```python
from build123d import *

# Parameters (mm, degrees)
F0_W         = 20
F0_H         = 47.7648153901
F1_DEPTH     = 3
F3_W         = 20
F3_H         = 23
F4_DEPTH     = 1.5
F5_T1_DEPTH  = 30.2867319519
F6_W         = 20
F6_H         = 2.1213203436
F7_DEPTH     = 7
F8_W         = 23.5785972327
F8_H         = 18.0557984859
F9_DEPTH     = 0.828
F10_SIZE     = 3
F11_R        = 2
F12_W        = 20
F12_H        = 16
F13_DEPTH    = 6
F14_T4_DEPTH = 61.5019292892
F14_T9_DEPTH = 61.5019292892
F15_R        = 2
F16_R        = 1
F17_W        = 2
F17_H        = 2
F18_DEPTH    = 3


# Not quite as in the source:
# - a fillet or chamfer that OpenCascade refuses, or shapes differently, is made with other operations: its cross-section is extruded or revolved along the edge and cut away or added


with BuildPart() as f1:
    # F0 (on Top) → F1 (new body)
    with BuildSketch(Plane.XY):
        Rectangle(F0_W, F0_H)
    extrude(amount=F1_DEPTH)

    # F3 (on offset) → F4 (join)
    with BuildSketch(Plane.XZ.offset(23.8824076951)):
        with Locations((0, -8.5)):
            Rectangle(F3_W, F3_H)
    extrude(amount=F4_DEPTH)

    # F5: chamfer of 2 on 1 edges, made by hand

    # F5_s2 → F5_t1 (cut)
    with BuildSketch(Plane.YZ.offset(-15.1433659759)):
        Polygon((-25.3824076951, -18), (-23.3824076951, -20), (-25.3824076951, -20), align=None)
    extrude(amount=F5_T1_DEPTH, mode=Mode.SUBTRACT)

    # F6 (on face) → F7 (join)
    with BuildSketch(Plane(origin=(0, -21.6912038475, -21.6912038475), x_dir=(1, 0, 0), z_dir=(0, -0.7071067812, -0.7071067812))):
        with Locations((0, 4.1594903709)):
            Rectangle(F6_W, F6_H)
    extrude(amount=F7_DEPTH)

    # F8 (on face) → F9 (cut)
    with BuildSketch(Plane(origin=(0, -2.1912038475, 2.1912038475), x_dir=(-1, 0, 0), z_dir=(0, 0.7071067812, -0.7071067812))):
        with Locations((-0.010414049, -33.0743109807)):
            Rectangle(F8_W, F8_H)
    extrude(amount=-F9_DEPTH, mode=Mode.SUBTRACT)

    # F10
    f10_edges = [f1.edges().sort_by_distance(p)[0] for p in [
        (-10, -29.874897, -23.407005),
        (10, -29.874897, -23.407005),
    ]]
    chamfer(f10_edges, length=F10_SIZE)

    # F11
    f11_edges = [f1.edges().sort_by_distance(p)[0] for p in [
        (0, -23.882408, 0),
        (0, -25.382408, -18),
        (0, -23.882408, -18.329031),
        (-10, -27.753577, -21.285685),
        (-7, -29.874897, -23.407005),
        (7, -29.874897, -23.407005),
        (10, -27.753577, -21.285685),
    ]]
    fillet(f11_edges, radius=F11_R)

    # F12 (on face) → F13 (join)
    with BuildSketch(Plane(origin=(0, 0, 0), x_dir=(1, 0, 0), z_dir=(0, 0, -1))):
        with Locations((0, 1.8824076951)):
            Rectangle(F12_W, F12_H)
    extrude(amount=F13_DEPTH)

    # F14: chamfer of 3 x 8 on 2 edges, made by hand


with BuildPart() as f14_tool2:
    # F14_s3 → F14_t4 (new body)
    with BuildSketch(Plane.YZ.offset(30.7509646446)):
        Polygon((-9.8824076951, 2), (-6.8824076951, -6), (-9.8824076951, -6), align=None)
    extrude(amount=-F14_T4_DEPTH)

    split(bisect_by=Plane.XY, keep=Keep.BOTTOM)


with BuildPart() as f1_1:
    add(f1.part)

    # F14_t1: cut F14_tool2
    add(f14_tool2.part, mode=Mode.SUBTRACT)


with BuildPart() as f14_tool7:
    # F14_s8 → F14_t9 (new body)
    with BuildSketch(Plane.YZ.offset(-30.7509646446)):
        Polygon((6.1175923049, 2), (3.1175923049, -6), (6.1175923049, -6), align=None)
    extrude(amount=F14_T9_DEPTH)

    split(bisect_by=Plane.XY, keep=Keep.BOTTOM)


with BuildPart() as f1_2:
    add(f1_1.part)

    # F14_t6: cut F14_tool7
    add(f14_tool7.part, mode=Mode.SUBTRACT)

    # F15
    f15_edges = [f1_2.edges().sort_by_distance(p)[0] for p in [
        (-10, 23.882408, 1.5),
        (10, 23.882408, 1.5),
    ]]
    fillet(f15_edges, radius=F15_R)

    # F16
    f16_edges = [f1_2.edges().sort_by_distance(p)[0] for p in [
        (-10, -1.882408, -6),
        (0, -6.882408, -6),
        (10, -1.882408, -6),
        (0, 3.117592, -6),
    ]]
    fillet(f16_edges, radius=F16_R)

    # F17 (on face) → F18 (cut, through all)
    with BuildSketch(Plane(origin=(0, 0, 0), x_dir=(1, 0, 0), z_dir=(0, 0, -1))):
        with Locations((-9, -6.3675923049)):
            Rectangle(F17_W, F17_H)
        with Locations((-9, 10.1324076951)):
            Rectangle(F17_W, F17_H)
    extrude(amount=-F18_DEPTH, mode=Mode.SUBTRACT)


solid = f1_2.part
```
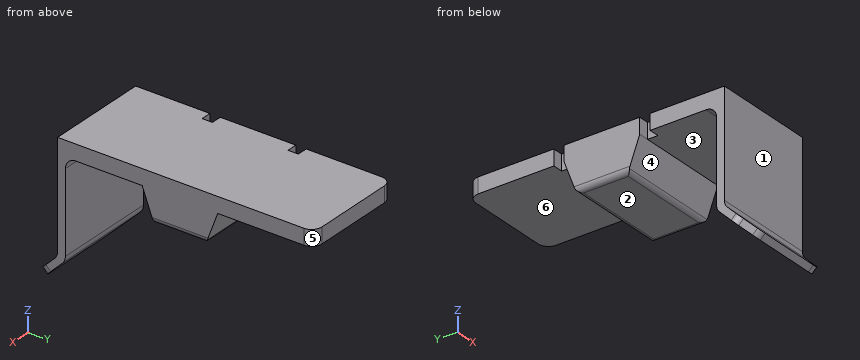
For this review, take the finished solid that the model builds, in its own axes (mm). Face numbers are marked on the shaded views. A direction names the side the tool comes from. Give positions to 0.01 mm unless a question says otherwise; leave off trailing zeros. Write each loop counter-clockwise with the first axis right and the second up, starting at its lowest first coordinate (ties: lowest second). Pieces come first, ordered by that corner, then holes. Notation, with made-up numbers: M 48,62 L 60,62 A29 ccw 60,88 Z; hole C 48,67.5 d8. An arc over 180 degrees is marked long. One line per item, written item: value.
1) Take a section at A-A, the plane y = -5.5. Write out the cut boundary in (x, z), then the cut area to 3 significant figures.
Results are:
outline: M -10,-5 A1 ccw -9,-6 L 9,-6 A1 ccw 10,-5 L 10,3 L -10,3 Z
area: 180 mm²
2) Take a section at B-B, the plane x = 4. Write out the cut boundary in (y, z).
Results are:
outline: M -30.33,-22.95 L -29.42,-23.86 L -24.47,-18.91 A2 ccw -23.88,-17.5 L -23.88,-2 A2 cw -21.88,0 L -9.13,0 L -7.13,-5.35 A1 ccw -6.19,-6 L 2.42,-6 A1 ccw 3.36,-5.35 L 5.37,0 L 23.88,0 L 23.88,3 L -25.38,3 L -25.38,-17.17 A2 cw -25.97,-18.59 Z
3) For the marked faces 1, 2 and 3, list the 3-axis set-ups (+Z, -Z, +X, -X, +Y, -Y) from which the entire face can be reached by the end or side of a thin tool; tool diameter is ignored.
Results are:
face 1: +Z, +X, -X, -Y
face 2: -Z, +X, -X, +Y
face 3: -Z, +X, -X
4) For P1, Ø1.5, axis at x = 6, y = 14, coming from the -Z side; P2, Ø4.5, axis at x = -2.5, y = -2.5, coming from the -Z side; P3, Ø0.6, axis at y = -10, z = 1, coming from the -X side, all flat-tipped, find the tip position at first contact; note any pin that passes through.
Results are:
P1: stops at z = 0
P2: stops at z = -6
P3: stops at x = -8
5) For line 1 (Z direction, x = 2.25, y = 2.5); line 2 (Z direction, x = 9, y = -20.5); line 3 (Y direction, x = -8, z = -4.5), list the stretches that pass through material, from the lowest coordinate up. Write a range as from..to.
Results are:
line 1: z = -6..3
line 2: z = 0..3
line 3: y = -25.38..-23.88, -7.44..3.68
6) Take a section at D-D, the plane y = -12. Write out the cut boundary in (x, z).
Results are:
outline: M -10,0 L 10,0 L 10,3 L -10,3 Z
7) Take a section at C-C, the plane z = 1.25. Write out the cut boundary in (x, y), then the cut area to 3 significant figures.
Results are:
outline: M -10,-25.38 L 10,-25.38 L 10,21.88 A2 ccw 8,23.88 L -8,23.88 A2 ccw -10,21.88 L -10,7.37 L -8,7.37 L -8,5.37 L -10,5.37 L -10,-9.13 L -8,-9.13 L -8,-11.13 L -10,-11.13 Z
area: 976 mm²
8) The part is to be moulded in two halves that separate along Y. For the marked faces 4, 5 and 6, say which applies: +Y half, -Y half, draft (parallel to the pull), parting line (faces both ways), or undercut.
Results are:
face 4: undercut
face 5: +Y half
face 6: draft
